Here's how the part is built. I have some questions about the finished solid (model axes, mm). A direction names the side the tool comes from. Give positions to 0.01 mm unless a question says otherwise; leave off trailing zeros. Write each loop counter-clockwise with the first axis right and the second up, starting at its lowest first coordinate (ties: lowest second). Pieces come first, ordered by that corner, then holes. Notation, with made-up numbers: (43.5, 75) -> (52.5, 75) arc R22 cw to (52.5, 98) -> close; hole circle Ø1 at (13, 68.25). An arc over 180 degrees is marked (long way). Put each result on its own line as item: value. Start each with the question number.
from build123d import *

# Parameters (mm, degrees)
F0_R     = 3.429
F1_DEPTH = 12.7
F2_W     = 6.096
F2_H     = 21.723506
F2_W_2   = 3.937
F2_H_2   = 13.240079
F3_DEPTH = 25.4
F4_W     = 7.366
F4_H     = 12.7
F5_DEPTH = 9.525
F6_R     = 2.63525
F7_DEPTH = 25.4


with BuildPart() as f1:
    # F0 (on Right) → F1 (new body)
    with BuildSketch(Plane.YZ):
        with BuildLine():
            ThreePointArc((0.913208, 3.069178), (3.228359, 0.820275), (6.35, 0))
            Line((6.35, 0), (44.45, 0))
            ThreePointArc((44.45, 0), (48.940128, 1.859872), (50.8, 6.35))
            ThreePointArc((50.8, 6.35), (48.940128, 10.840128), (44.45, 12.7))
            Line((44.45, 12.7), (0, 12.7))
            Line((0, 12.7), (-1.27, 12.7))
            Line((-1.27, 12.7), (0.913208, 3.069178))
        make_face()
        with Locations((6.35, 6.35)):
            Circle(F0_R, mode=Mode.SUBTRACT)
        with Locations((44.45, 6.35)):
            Circle(F0_R, mode=Mode.SUBTRACT)
    extrude(amount=F1_DEPTH)

    # F2 (on face) → F3 (cut)
    with BuildSketch(Plane.XY.offset(12.7)):
        with Locations((6.35, 1.635321)):
            Rectangle(F2_W, F2_H)
        with Locations((1.9685, 44.466039)):
            Rectangle(F2_W_2, F2_H_2)
        with Locations((10.7315, 44.466039)):
            Rectangle(F2_W_2, F2_H_2)
    extrude(amount=-F3_DEPTH, mode=Mode.SUBTRACT)

    # F4 (on face) → F5 (cut)
    with BuildSketch(Plane.YZ.offset(12.7)):
        with Locations((25.4, 6.35)):
            Rectangle(F4_W, F4_H)
    extrude(amount=-F5_DEPTH, mode=Mode.SUBTRACT)

    # F6 (on face) → F7 (cut)
    with BuildSketch(Plane.YZ.offset(3.175)):
        with Locations((25.291821, 6.35)):
            Circle(F6_R)
    extrude(amount=-F7_DEPTH, mode=Mode.SUBTRACT)


solid = f1.part
1) I'm going to push flat-ended pins straight in: pin 1 Ø4 at (y, z) = (42, 6.5) entering from +X; pin 2 Ø1.2 at (x, z) = (1, 7.5) entering from +Y; pin 3 Ø5 at (x, z) = (4, 3) entering from +Y. Where does each tip first touch, or does it pass through?
2) I want a section at C-C, the plane z = 5.25. State how many separate pieces and enclosed holes the cut face has, and give its area (3 significant figures).
3) I want a section at B-B, the plane y = 9. Write out the boundary of the cut face in (x, z), and give its area (3 significant figures).
4) Which directions (+Z, -Z, +X, -X, +Y, -Y) give clear straight access to the entire face, cutting with the end or side of a thin tool? Please do faces 5 (the flat face through (11, 37.846, 6)), 6 (the flat face through (6.3, 29.4, 0)), 7 (the flat face through (3.175, 25.3, 9.3)).
5) I want a section at D-D, the plane x = 1.25. Write out the boundary of the cut face in (y, z).
6) I need wall thicknesses on probe 1 along Y at (x, z) = (5.6, 6.35); probe 2 along Y at (x, z) = (5.75, 7.75); probe 3 along X at (y, z) = (2, 3.25). Which ranges of each line are inside material? Lowest first, please.
7) Thinking about a two-plate mould opening in X: for faces 1 (the flat face through (0, 18, 6)), 2 (the flat face through (3.302, 9, 9)), 3 (the cylindrical face through (11.03, 3.19, 0.84)), 4 (the flat face through (6, 12.497, 6)), which applies, released by +X, released by -X, zero draft, split by the parting line, or undercut?
8) I want a section at A-A, the plane x = 11.5. Write out the boundary of the cut face in (y, z), and give its area (3 significant figures).
Established:
1. pin 1: stops at x = 8.76
1. pin 2: stops at y = 37.85
1. pin 3: stops at y = 50.74
2. separate pieces: 5
2. enclosed holes: 0
2. area: 304 mm2
3. outline: (0, 0) -> (3.3, 0) -> (3.3, 4.17) -> (0, 4.17) -> close; (0, 8.53) -> (3.3, 8.53) -> (3.3, 12.7) -> (0, 12.7) -> close; (9.4, 0) -> (12.7, 0) -> (12.7, 4.17) -> (9.4, 4.17) -> close; (9.4, 8.53) -> (12.7, 8.53) -> (12.7, 12.7) -> (9.4, 12.7) -> close
3. area: 55.1 mm2
4. face 5: +Z, -Z, +X, +Y
4. face 6: -Z, +X, -X, +Y, -Y
4. face 7: +Z, -Z, +X
5. outline: (-1.27, 12.7) -> (0.91, 3.07) arc R6.35 ccw to (6.35, 0) -> (37.85, 0) -> (37.85, 12.7) -> close; hole circle Ø6.86 at (6.35, 6.35); hole circle Ø5.27 at (25.29, 6.35)
6. probe 1: y = 12.5 to 21.72, 29.08 to 41.02, 47.88 to 50.8
6. probe 2: y = 12.5 to 21.72, 29.08 to 41.32, 47.58 to 50.64
6. probe 3: x = 0 to 3.3, 9.4 to 12.7
7. face 1: released by -X
7. face 2: undercut
7. face 3: zero draft
7. face 4: undercut
8. outline: (-1.27, 12.7) -> (0.91, 3.07) arc R6.35 ccw to (6.35, 0) -> (21.72, 0) -> (21.72, 12.7) -> close; (29.08, 0) -> (37.85, 0) -> (37.85, 12.7) -> (29.08, 12.7) -> close; hole circle Ø6.86 at (6.35, 6.35)
8. area: 344 mm2
